Check sheet for the modelled part. Datum: model origin and axes. Units: mm. Face numbers are marked on the shaded views. A direction names the side the tool comes from. Round coordinates to 2 decimals unless told otherwise and drop trailing zeros. Write each loop counter-clockwise with the first axis right and the second up, starting at its lowest first coordinate (ties: lowest second). Pieces come first, ordered by that corner, then holes. Notation, with made-up numbers: (67, -14) -> (96, -14) arc R19 ccw to (96, 18) -> close; hole circle Ø3 at (46.25, -33). An arc over 180 degrees is marked (long way). One line per item, written item: value.
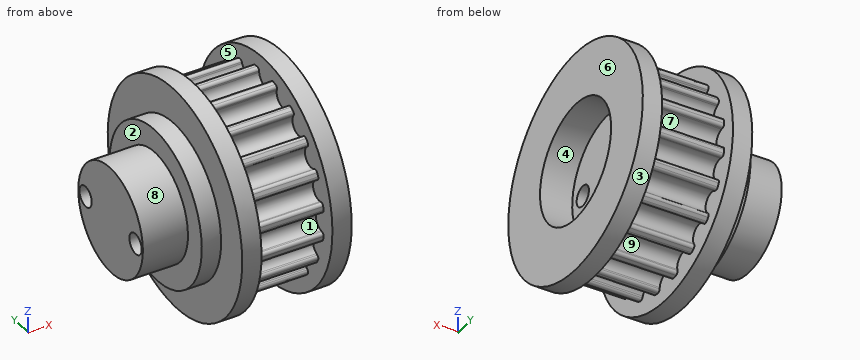
from build123d import *

# Parameters (mm, degrees)
CHAMFER_1_SIZE           = 1
SKETCH_4_W               = 2
SKETCH_4_H               = 1
CUT_EXTRUDE_1_DEPTH      = 36.4233722
CUT_EXTRUDE_2_REACH      = 37.423
PATTERN_CIRCULAR_3_COUNT = 20
SKETCH_8_R               = 17.530868232
CUT_EXTRUDE_3_DEPTH      = 17
SKETCH_9_R               = 7.01145328
EXTRUDE_1_DEPTH          = 11
SKETCH_10_R              = 17.5
EXTRUDE_2_DEPTH          = 3
EXTRUDE_START            = 3
SKETCH_11_R              = 17.5
EXTRUDE_3_DEPTH          = 3
SKETCH_12_R              = 9.25
CUT_EXTRUDE_4_DEPTH      = 5
SKETCH_13_R              = 1.6
CUT_EXTRUDE_5_DEPTH      = 28.504545079
SKETCH_14_R              = 12
SKETCH_14_R_2            = 3.5
SKETCH_14_R_3            = 1.6
EXTRUDE_4_DEPTH          = 3
SKETCH_17_R              = 8.4
EXTRUDE_6_DEPTH          = 7
SKETCH_18_R              = 1.6
CUT_EXTRUDE_7_DEPTH      = 34.11344138


with BuildPart() as part:
    # 草图1 → 旋转1 (revolve)
    with BuildSketch(Plane.XY, mode=Mode.PRIVATE) as revolve_1_sk:
        Polygon((0, 3.0686), (0, 15.343), (28, 15.343), (28, 6.1372), (20, 6.1372), (20, 3.0686), align=None)
    revolve(revolve_1_sk.sketch.rotate(Axis((0, 0, 0), (1, 0, 0)), 90), axis=Axis((0, 0, 0), (1, 0, 0)))

    # 倒角1
    chamfer_1_edges = [part.edges().sort_by_distance(p)[0] for p in [
        (20, 0, -3.0686),
        (0, 0, -3.0686),
    ]]
    chamfer(chamfer_1_edges, length=CHAMFER_1_SIZE)

    # 草图4 → 切除-拉伸1 (cut, through all)
    with BuildSketch(Plane.ZY):
        with Locations((0, 3.401087031)):
            Rectangle(SKETCH_4_W, SKETCH_4_H)
    extrude(amount=-CUT_EXTRUDE_1_DEPTH, mode=Mode.SUBTRACT)

    # 草图6 → 切除-拉伸2 (cut, up to next)
    with BuildSketch(Plane(origin=(0, 0, 0), x_dir=(0, 0, -1), z_dir=(1, 0, 0)), mode=Mode.PRIVATE) as cut_extrude_2_sk1:
        with BuildLine():
            Line((1.576146133, 14.779086011), (1.548371997, 14.552883824))
            ThreePointArc((1.548371997, 14.552883824), (0, 13.183), (-1.548371997, 14.552883824))
            Line((-1.548371997, 14.552883824), (-1.576146133, 14.779086011))
            ThreePointArc((-1.576146133, 14.779086011), (-1.760156371, 15.101239842), (-2.118855897, 15.195989559))
            ThreePointArc((-2.118855897, 15.195989559), (-2.356297075, 15.160986547), (-2.593161675, 15.122273689))
            Line((-2.593161675, 15.122273689), (-6.402553611, 46.147281297))
            ThreePointArc((-6.402553611, 46.147281297), (0, 46.589314911), (6.402553611, 46.147281297))
            Line((6.402553611, 46.147281297), (2.593161675, 15.122273689))
            ThreePointArc((2.593161675, 15.122273689), (2.356297075, 15.160986547), (2.118855897, 15.195989559))
            ThreePointArc((2.118855897, 15.195989559), (1.760156371, 15.101239842), (1.576146133, 14.779086011))
        make_face()
    cut_extrude_2_tool1 = extrude(cut_extrude_2_sk1.sketch, amount=CUT_EXTRUDE_2_REACH, mode=Mode.PRIVATE) & part.part
    cut_extrude_2 = cut_extrude_2_tool1.solids().sort_by_distance((0, 32.67982, 0))[0]
    add(cut_extrude_2, mode=Mode.SUBTRACT)

    # 阵列(圆周)3: 切除-拉伸2 ×20 about axis
    pattern_circular_3_axis = Axis((0, 0, 0), (1, 0, 0))
    for i in range(1, PATTERN_CIRCULAR_3_COUNT):
        add(cut_extrude_2.rotate(pattern_circular_3_axis, i * 360 / PATTERN_CIRCULAR_3_COUNT), mode=Mode.SUBTRACT)

    # 草图8 → 切除-拉伸3 (cut)
    with BuildSketch(Plane(origin=(28, 0, 0), x_dir=(0, 0, -1), z_dir=(1, 0, 0))):
        Circle(SKETCH_8_R)
    extrude(amount=-CUT_EXTRUDE_3_DEPTH, mode=Mode.SUBTRACT)

    # 草图9 → 凸台-拉伸1 (add)
    with BuildSketch(Plane(origin=(11, 0, 0), x_dir=(0, 0, -1), z_dir=(1, 0, 0))):
        Circle(SKETCH_9_R)
    extrude(amount=-EXTRUDE_1_DEPTH)

    # 草图10 → 凸台-拉伸2 (add)
    with BuildSketch(Plane(origin=(11, 0, 0), x_dir=(0, 0, -1), z_dir=(1, 0, 0))):
        Circle(SKETCH_10_R)
    extrude(amount=EXTRUDE_2_DEPTH)

    # 草图11 → 凸台-拉伸3 (add)
    with BuildSketch(Plane.ZY.offset(EXTRUDE_START)):
        with Locations(Location((0, 0, 0), (0, 0, 180))):
            Circle(SKETCH_11_R)
    extrude(amount=-EXTRUDE_3_DEPTH)

    # 草图12 → 切除-拉伸4 (cut)
    with BuildSketch(Plane(origin=(14, 0, 0), x_dir=(0, 0, -1), z_dir=(1, 0, 0))):
        Circle(SKETCH_12_R)
    extrude(amount=-CUT_EXTRUDE_4_DEPTH, mode=Mode.SUBTRACT)

    # 草图13 → 切除-拉伸5 (cut, through all)
    with BuildSketch(Plane(origin=(9, 0, 0), x_dir=(0, 0, -1), z_dir=(1, 0, 0))):
        with Locations((0, 6.5)):
            Circle(SKETCH_13_R)
        with Locations((0, -6.5)):
            Circle(SKETCH_13_R)
    extrude(amount=-CUT_EXTRUDE_5_DEPTH, mode=Mode.SUBTRACT)

    # 草图14 → 凸台-拉伸4 (add)
    # profile 1 of 3: a face of its own
    with BuildSketch(Plane.ZY.offset(3)):
        Circle(SKETCH_14_R)
        with Locations((0, -6.5)):
            Circle(SKETCH_14_R_2, mode=Mode.SUBTRACT)
        with Locations((0, 6.5)):
            Circle(SKETCH_14_R_2, mode=Mode.SUBTRACT)
    # profile 2 of 3: a face of its own
    with BuildSketch(Plane.ZY.offset(3)):
        with Locations((0, 6.5)):
            Circle(SKETCH_14_R_2)
        with Locations(Location((0, 6.5, 0), (0, 0, 180))):
            Circle(SKETCH_14_R_3, mode=Mode.SUBTRACT)
    # profile 3 of 3: a face of its own
    with BuildSketch(Plane.ZY.offset(3)):
        with Locations((0, -6.5)):
            Circle(SKETCH_14_R_2)
        with Locations(Location((0, -6.5, 0), (0, 0, 180))):
            Circle(SKETCH_14_R_3, mode=Mode.SUBTRACT)
    extrude(amount=EXTRUDE_4_DEPTH)

    # 草图17 → 凸台-拉伸6 (add)
    with BuildSketch(Plane.ZY.offset(6)):
        Circle(SKETCH_17_R)
    extrude(amount=EXTRUDE_6_DEPTH)

    # 草图18 → 切除-拉伸7 (cut, through all)
    with BuildSketch(Plane(origin=(9, 0, 0), x_dir=(0, 0, -1), z_dir=(1, 0, 0))):
        with Locations((0, 6.5)):
            Circle(SKETCH_18_R)
        with Locations((0, -6.5)):
            Circle(SKETCH_18_R)
    extrude(amount=-CUT_EXTRUDE_7_DEPTH, mode=Mode.SUBTRACT)


solid = part.part
Item 1: Sectioned sample at C-C on y = 0. Enter the section's corners in (x, z).
Answer:
outline: (-13, -8.4) -> (-6, -8.4) -> (-6, -12) -> (-3, -12) -> (-3, -17.5) -> (0, -17.5) -> (0, -13.18) -> (11, -13.18) -> (11, -17.5) -> (14, -17.5) -> (14, -9.25) -> (9, -9.25) -> (9, 9.25) -> (14, 9.25) -> (14, 17.5) -> (11, 17.5) -> (11, 13.18) -> (0, 13.18) -> (0, 17.5) -> (-3, 17.5) -> (-3, 12) -> (-6, 12) -> (-6, 8.4) -> (-13, 8.4) -> close
Item 2: Depth check by flat-ended pin: P1, Ø4, axis at x = 8, y = -0.5, coming from the -Z side; P2, Ø2, axis at x = 2, z = -13, coming from the -Y side; P3, Ø2.5, axis at y = -6.5, z = 0, coming from the +X side; P4, Ø5, axis at x = 8, z = 3, coming from the +Y side. Enter the tip coordinate at first touch or a pass-through.
Answer:
P1: stops at z = -15.2
P2: stops at y = -7.47
P3: passes through
P4: stops at y = 15.2
Item 3: Sectioned sample at B-B on x = -2. Enter the section's corners in (y, z).
Answer:
outline: circle Ø35 at (0, 0); hole circle Ø3.2 at (-6.5, 0); hole circle Ø3.2 at (6.5, 0)
Item 4: Mould release check, pull along Z, two halves, no side actions. Record for the marked faces 6, 7, 8 and 9: pulls with the +Z half, pulls with the -Z half, needs draft (parallel to the pull), parting line crosses it, or undercut.
Answer:
face 6: needs draft
face 7: undercut
face 8: parting line crosses it
face 9: undercut
Item 5: Tool access check on the marked faces 1, 2, 3, 4 and 5. Record the directions out of +Z, -Z, +X, -X, +Y, -Y that give a thin tool (end or side, any length) a straight path to the whole face; none if there is none.
Answer:
face 1: -Y
face 2: -X
face 3: +X, -X
face 4: +X
face 5: none
Item 6: Thickness scan on line 1 (Y direction, x = 1.75, z = 0); line 2 (X direction, y = -8, z = 14); line 3 (Z direction, x = 0.5, y = -13). Record the ranges inside material, lowest first.
Answer:
line 1: y = -13.18 to -8.1, -4.9 to 4.9, 8.1 to 13.18
line 2: x = -3 to 0, 11 to 14
line 3: z = -7.46 to -5.73, -3.38 to 3.38, 5.73 to 7.46
Item 7: Sectioned sample at A-A on z = 0. Count the separate pieces of the cut face and the enclosed holes in it, and give its area (3 significant figures).
Answer:
separate pieces: 3
enclosed holes: 0
area: 456 mm^2
